Here's how the part is built. I have some questions about the finished solid (model axes, mm). A direction names the side the tool comes from. Round coordinates to 2 decimals unless told otherwise and drop trailing zeros. Use one line per item in the form item = value. Start each with the question number.
```python
from build123d import *

# Parameters (mm, degrees)
CUT_EXTRUDE1_START  = -3
CUT_EXTRUDE1_DEPTH  = 12
CIRPATTERN1_COUNT   = 10
BOSS_EXTRUDE1_START = 10.5
SKETCH7_R           = 2.383452373
SKETCH7_R_2         = 1.5
BOSS_EXTRUDE1_DEPTH = 21


with BuildPart() as part:
    # Sketch6 → Revolve1 (revolve)
    with BuildSketch(Plane.XY):
        with BuildLine():
            Line((9.75, 10), (10.5, 10))
            Line((10.5, 10), (10.5, 2))
            Line((10.5, 2), (-10.5, 2))
            Line((-10.5, 2), (-10.5, 4))
            Line((-10.5, 4), (-4.5, 4))
            Line((-4.5, 4), (-4.5, 10))
            Line((-4.5, 10), (-3.75, 10))
            ThreePointArc((-3.75, 10), (-3.191617437, 8.818070474), (-3, 7.525))
            Line((-3, 7.525), (9, 7.525))
            ThreePointArc((9, 7.525), (9.191617437, 8.818070474), (9.75, 10))
        make_face()
    revolve(axis=Axis((-10.5, 0, 0), (1, 0, 0)))

    # Sketch3 → Cut-Extrude1 (cut)
    with BuildSketch(Plane(origin=(0, 0, 0), x_dir=(0, 0, -1), z_dir=(1, 0, 0)).offset(CUT_EXTRUDE1_START)):
        with BuildLine():
            Line((-1.325, 7.407428704), (-0.907223869, 6.259598218))
            Line((-0.907223869, 6.259598218), (0.907223869, 6.259598218))
            Line((0.907223869, 6.259598218), (1.325, 7.407428704))
            ThreePointArc((1.325, 7.407428704), (0, 7.525), (-1.325, 7.407428704))
        make_face()
    cut_extrude1 = extrude(amount=CUT_EXTRUDE1_DEPTH, mode=Mode.SUBTRACT)

    # CirPattern1: Cut-Extrude1 ×10 about axis
    cirpattern1_axis = Axis((0, 0, 0), (1, 0, 0))
    for i in range(1, CIRPATTERN1_COUNT):
        add(cut_extrude1.rotate(cirpattern1_axis, i * 360 / CIRPATTERN1_COUNT), mode=Mode.SUBTRACT)

    # Sketch7 → Boss-Extrude1 (add)
    with BuildSketch(Plane(origin=(0, 0, 0), x_dir=(0, 0, -1), z_dir=(1, 0, 0)).offset(BOSS_EXTRUDE1_START)):
        Circle(SKETCH7_R)
        Circle(SKETCH7_R_2, mode=Mode.SUBTRACT)
    extrude(amount=-BOSS_EXTRUDE1_DEPTH)


solid = part.part
```
1) If we mould it in two halves opening along Z, with no side actions, what happens to faces 5 (the flat face through (2.92, -3.18, 6.16)), 6 (the flat face through (9, 6, -4)), 7 (the flat face through (-4.5, -4.3, 0.1))? For each: +Z half, -Z half, draft (parallel to the pull), parting line (faces both ways), or undercut.
2) Will these pins go through, and if not, where does the flat tip stop? pin 1 Ø1.5 at (x, z) = (-3.5, 7) entering from -Y; pin 2 Ø0.7 at (y, z) = (6, 4.5) entering from -X; pin 3 Ø1.5 at (x, y) = (3.5, -7) entering from +Z.
3) If I drill on line 1 (Y direction, x = -0.75, z = 0); line 2 (X direction, y = 1.5, z = 7.5); line 3 (X direction, y = 5, z = -0.75), over which ranges is the centre line in solid material (lowest first)?
4) On a 3-axis mill with a long thin cutter (end or side, diameter ignored), from which of +Z, -Z, +X, -X, +Y, -Y can I reach the whole of each face in a straight line? I mean faces 1 (the cylindrical face through (3.08, -7.15, 2.34)), 2 (the cylindrical face through (3.084, -4.435, -6.079)), 3 (the flat face through (2.92, 3.17, 6.15)), 4 (the flat face through (2.916, -6.825, 1.113)). Say none if no direction works.
Completed:
q1.face_5 = +Z half
q1.face_6 = undercut
q1.face_7 = draft
q2.pin_1 = -7.77
q2.pin_2 = -4.5
q2.pin_3 = 3.28
q3.line_1 = -6.26 to -1.5, 1.5 to 6.26
q3.line_2 = -4.5 to -3, 9 to 10.5
q3.line_3 = -4.5 to 10.5
q4.face_1 = +Z, -Y
q4.face_2 = -Z, -Y
q4.face_3 = +Z
q4.face_4 = -Y
